Work out the finished part from the listing and answer in its coordinate system (mm). Round coordinates to 2 decimals unless told otherwise and drop trailing zeros. Write each loop counter-clockwise with the first axis right and the second up, starting at its lowest first coordinate (ties: lowest second). Pieces come first, ordered by that corner, then holes. Notation, with made-up numbers: (-0.5, 55.25) - (51.5, 55.25) arc R30 cw to (51.5, 82.25) - close; hole circle Ø6 at (86.5, -15). An arc over 180 degrees is marked (long way). Answer as a JSON object with one key per item and string values.
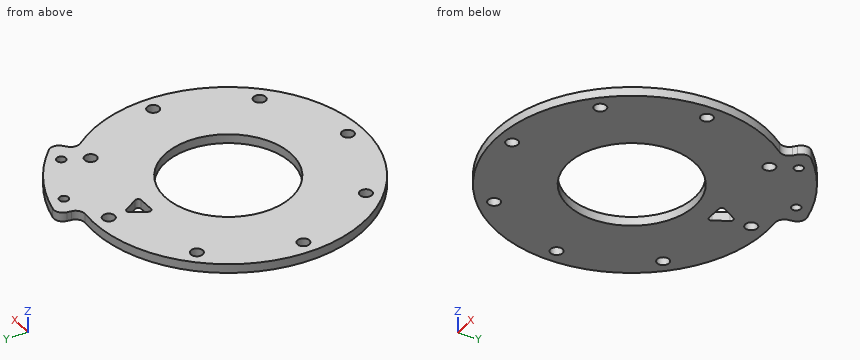
```python
from build123d import *

# Parameters (mm, degrees)
SKETCH_1_R          = 45
SKETCH_1_R_2        = 21
EXTRUDE_1_DEPTH     = 3
SKETCH_2_R          = 2
CUT_EXTRUDE_1_DEPTH = 10
CUT_EXTRUDE_2_DEPTH = 3
EXTRUDE_START       = -3
SKETCH_3_R          = 1.5
EXTRUDE_3_DEPTH     = 3
FILLET_2_R          = 1
FILLET_3_R          = 3


with BuildPart() as part:
    # 草图1 → 凸台-拉伸1 (new body)
    with BuildSketch(Plane.XY):
        Circle(SKETCH_1_R)
        Circle(SKETCH_1_R_2, mode=Mode.SUBTRACT)
    extrude(amount=EXTRUDE_1_DEPTH)

    # 草图2 → 切除-拉伸1 (cut)
    with BuildSketch(Plane.XY.offset(3)):
        with Locations((0, 40)):
            Circle(SKETCH_2_R)
        with Locations((28.284271247, 28.284271247)):
            Circle(SKETCH_2_R)
        with Locations((40, 0)):
            Circle(SKETCH_2_R)
        with Locations((28.284271247, -28.284271247)):
            Circle(SKETCH_2_R)
        with Locations((0, -40)):
            Circle(SKETCH_2_R)
        with Locations((-28.284271247, -28.284271247)):
            Circle(SKETCH_2_R)
        with Locations((-40, 0)):
            Circle(SKETCH_2_R)
        with Locations((-28.284271247, 28.284271247)):
            Circle(SKETCH_2_R)
    extrude(amount=-CUT_EXTRUDE_1_DEPTH, mode=Mode.SUBTRACT)

    # 草图4 → 切除-拉伸2 (cut)
    with BuildSketch(Plane.XY.offset(3)):
        Polygon((4.330127019, 27.5), (0, 35), (-4.330127019, 27.5), align=None)
    extrude(amount=-CUT_EXTRUDE_2_DEPTH, mode=Mode.SUBTRACT)

    # 草图3 → 凸台-拉伸3 (add)
    with BuildSketch(Plane.XY.offset(3).offset(EXTRUDE_START)):
        with BuildLine():
            Line((9.116529328, 51.702407033), (7.814167995, 44.316348886))
            ThreePointArc((7.814167995, 44.316348886), (22.5, 38.97114317), (34.47199994, 28.925442436))
            Line((34.47199994, 28.925442436), (40.217333264, 33.746349509))
            ThreePointArc((40.217333264, 33.746349509), (26.25, 45.466333699), (9.116529328, 51.702407033))
        make_face()
        with Locations((32.160254038, 35.703193978)):
            Circle(SKETCH_3_R, mode=Mode.SUBTRACT)
        with Locations((14.839745962, 45.703193978)):
            Circle(SKETCH_3_R, mode=Mode.SUBTRACT)
    extrude(amount=EXTRUDE_3_DEPTH)

    # 圆角2
    fillet_2_edges = [part.edges().sort_by_distance(p)[0] for p in [
        (4.330127019, 27.5, 1.5),
        (-4.330127019, 27.5, 1.5),
        (0, 35, 1.5),
    ]]
    fillet(fillet_2_edges, radius=FILLET_2_R)

    # 圆角3
    fillet_3_edges = [part.edges().sort_by_distance(p)[0] for p in [
        (40.217333264, 33.746349509, 1.5),
        (34.47199994, 28.925442436, 1.5),
        (7.814167995, 44.316348886, 1.5),
        (9.116529328, 51.702407033, 1.5),
    ]]
    fillet(fillet_3_edges, radius=FILLET_3_R)


solid = part.part
```
Item 1: A cutting plane is placed at D-D (x = 25). Write down the section's boundary in (y, z), and give its area (3 significant figures).
Results found:
{"outline": "(-37.42, 0) - (46.17, 0) - (46.17, 3) - (-37.42, 3) - close", "area": "251 mm²"}
Item 2: A cutting plane is placed at B-B (x = 40). Write down the section's boundary in (y, z).
Results found:
{"outline": "(-20.62, 0) - (-2, 0) - (-2, 3) - (-20.62, 3) - close; (2, 0) - (20.62, 0) - (20.62, 3) - (2, 3) - close"}
Item 3: Consider line 1 along Y through (x, z) = (0, 1.1); line 2 along X through (y, z) = (-28.5, 2.85); line 3 along X through (y, z) = (-27, 2.8). Determine where each line is inside the solid, lowest interval first.
Results found:
{"line 1": "-45 to -42, -38 to -21, 21 to 27.5, 34 to 38, 42 to 45", "line 2": "-34.82 to -30.27, -26.3 to 26.3, 30.27 to 34.82", "line 3": "-36 to -29.82, -26.75 to 26.75, 29.82 to 36"}
Item 4: This flat-tipped pin is pushed along its axis until it touches: P1, Ø1, axis at y = 37, z = 0.5, coming from the -X side. Where does it stop, or does it pass through?
Results found:
{"P1": "x = -26.32"}
Item 5: A cutting plane is placed at C-C (z = 0.8). Give the number of separate pieces and of enclosed holes in the cut face, and give its area (3 significant figures).
Results found:
{"separate pieces": "1", "enclosed holes": "12", "area": "5,090 mm²"}
Item 6: A cutting plane is placed at A-A (y = 4.5). Write down the section's boundary in (x, z), and give its area (3 significant figures).
Results found:
{"outline": "(-44.77, 0) - (-20.51, 0) - (-20.51, 3) - (-44.77, 3) - close; (20.51, 0) - (44.77, 0) - (44.77, 3) - (20.51, 3) - close", "area": "146 mm²"}
